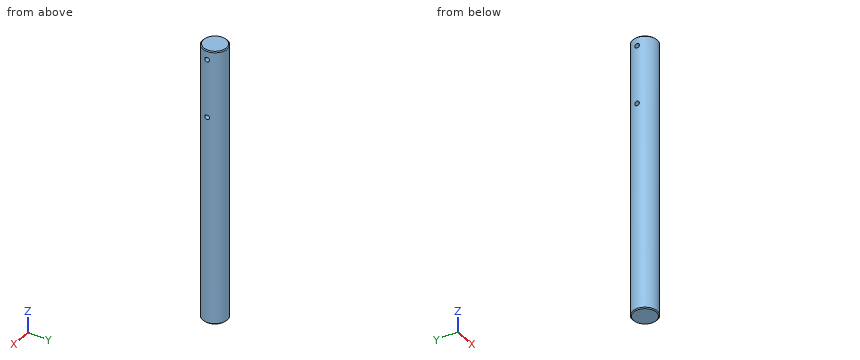
```python
from build123d import *

# Parameters (mm, degrees)
SKETCH1_W               = 90
SKETCH1_H               = 4
CHAMFER1_SIZE           = 0.3
CUT_EXTRUDE1_DEPTH      = 46.354161882
CUT_EXTRUDE1_DEPTH_BACK = 46.354161882
SKETCH6_R               = 0.75


with BuildPart() as part:
    # Sketch1 → Revolve1 (revolve)
    with BuildSketch(Plane(origin=(0, 0, 0), x_dir=(0, 0, -1), z_dir=(1, 0, 0)), mode=Mode.PRIVATE) as revolve1_sk:
        with Locations((0, 2)):
            Rectangle(SKETCH1_W, SKETCH1_H)
    revolve(revolve1_sk.sketch.rotate(Axis((0, 0, 0), (0, 0, -1)), 90), axis=Axis((0, 0, 0), (0, 0, -1)))

    # Chamfer1
    chamfer1_edges = [part.edges().sort_by_distance(p)[0] for p in [
        (-4, 0, 45),
        (-4, 0, -45),
    ]]
    chamfer(chamfer1_edges, length=CHAMFER1_SIZE)

    # Sketch6 → Cut-Extrude1 (cut, two sides: drawn at the far end of the back side and taken through both)
    with BuildSketch(Plane(origin=(0, 0, 0), x_dir=(0, 0, -1), z_dir=(1, 0, 0)).offset(-CUT_EXTRUDE1_DEPTH_BACK)):
        with Locations((-23, 0)):
            Circle(SKETCH6_R)
        with Locations((-42, 0)):
            Circle(SKETCH6_R)
    extrude(amount=CUT_EXTRUDE1_DEPTH + CUT_EXTRUDE1_DEPTH_BACK, mode=Mode.SUBTRACT)


solid = part.part
```
For this review, take the finished solid that the model builds, in its own axes (mm). Round coordinates to 2 decimals unless told otherwise and drop trailing zeros. Order: outer loops, then holes, each group sorted by start corner. A loop starts at its lowest first (then second) coordinate and runs counter-clockwise, first axis right, second up.
Q1. We need section C-C, the plane x = 2.25. State how many separate pieces and enclosed holes the cut face has, plus the area to 3 significant figures.
Findings below:
separate pieces: 1
enclosed holes: 2
area: 592 mm2
Q2. We need section A-A, the plane z = -2. Give the boundary of the cut face in (x, y).
Findings below:
outline: circle Ø8 at (0, 0)
Q3. We need section B-B, the plane z = 42. Give the boundary of the cut face in (x, y).
Findings below:
outline: (-3.93, -0.75) arc R4 ccw to (3.93, -0.75) - close; (-3.93, 0.75) - (3.93, 0.75) arc R4 ccw to start
Q4. Wall thickness on line 1 (Z direction, x = -2, y = 0); line 2 (Y direction, x = 0.75, z = 42); line 3 (X direction, y = -1.5, z = 39.5): over which ranges is each line inside the solid? List them lowest first.
Findings below:
line 1: z = -45 to 22.25, 23.75 to 41.25, 42.75 to 45
line 2: y = -3.93 to -0.75, 0.75 to 3.93
line 3: x = -3.71 to 3.71
Q5. Insertion check: P1, Ø1.2, axis at y = 0, z = 23, coming from the -X side; P2, Ø1, axis at x = -2, z = 35, coming from the -Y side; P3, Ø4, axis at y = 2.5, z = 9, coming from the +X side. Each pin has a flat end and moves straight along its axis. Give the tip position at first contact, or say it passes through.
Findings below:
P1: passes through
P2: stops at y = -3.71
P3: stops at x = 3.97
